Could you check a few things on this model? Use its own coordinates, in mm. A direction names the side the tool comes from. Give positions to 0.01 mm unless a question says otherwise; leave off trailing zeros. Write each loop counter-clockwise with the first axis right and the second up, starting at its lowest first coordinate (ties: lowest second). Pieces come first, ordered by that corner, then holes. Notation, with made-up numbers: M 30,89 L 61,89 A27 ccw 61,121 Z; hole C 9,47.25 d8. An arc over 180 degrees is marked long. One line per item, written item: value.
```python
from build123d import *

# Parameters (mm, degrees)
SKETCH1_R           = 10
BOSS_EXTRUDE1_DEPTH = 6
BOSS_EXTRUDE2_DEPTH = 6
CIRPATTERN1_COUNT   = 24
SKETCH3_R           = 12.65
SKETCH3_R_2         = 12
CUT_EXTRUDE1_DEPTH  = 6
CUT_EXTRUDE2_DEPTH  = 6
SKETCH5_R           = 1.5
CUT_EXTRUDE3_DEPTH  = 6
BOSS_EXTRUDE3_DEPTH = 6


with BuildPart() as part:
    # Sketch1 → Boss-Extrude1 (new body)
    with BuildSketch(Plane.XY):
        Circle(SKETCH1_R)
    extrude(amount=BOSS_EXTRUDE1_DEPTH)

    # Sketch2 → Boss-Extrude2 (add)
    with BuildSketch(Plane.XY):
        with BuildLine():
            Line((0, 12.65), (-0.9, 9.959417654))
            ThreePointArc((-0.9, 9.959417654), (0, 10), (0.9, 9.959417654))
            Line((0.9, 9.959417654), (0, 12.65))
        make_face()
    boss_extrude2 = extrude(amount=BOSS_EXTRUDE2_DEPTH)

    # CirPattern1: Boss-Extrude2 ×24 about axis
    cirpattern1_axis = Axis((0, 0, 0), (0, 0, 1))
    for i in range(1, CIRPATTERN1_COUNT):
        add(boss_extrude2.rotate(cirpattern1_axis, i * 360 / CIRPATTERN1_COUNT))

    # Sketch3 → Cut-Extrude1 (cut)
    with BuildSketch(Plane.XY):
        Circle(SKETCH3_R)
        Circle(SKETCH3_R_2, mode=Mode.SUBTRACT)
    extrude(amount=CUT_EXTRUDE1_DEPTH, mode=Mode.SUBTRACT)

    # Sketch4 → Cut-Extrude2 (cut)
    with BuildSketch(Plane.XY):
        with BuildLine():
            Line((0, 0), (0, 12))
            ThreePointArc((0, 12), (11.769423365, -2.341083864), (-4.592201188, -11.08655439))
            Line((-4.592201188, -11.08655439), (-3.826834324, -9.238795325))
            Line((-3.826834324, -9.238795325), (0, 0))
        make_face()
    extrude(amount=CUT_EXTRUDE2_DEPTH, mode=Mode.SUBTRACT)

    # Sketch5 → Cut-Extrude3 (cut)
    with BuildSketch(Plane.XY):
        Circle(SKETCH5_R)
    extrude(amount=CUT_EXTRUDE3_DEPTH, mode=Mode.SUBTRACT)

    # Sketch6 → Boss-Extrude3 (add)
    with BuildSketch(Plane.XY):
        with BuildLine():
            Line((0, 1.5), (0, 12))
            Line((0, 12), (7, 12))
            Line((7, 12), (7, 9.904493766))
            Line((7, 9.904493766), (11, 9.904493766))
            Line((11, 9.904493766), (11, -10.095506234))
            Line((11, -10.095506234), (7, -10.095506234))
            Line((7, -10.095506234), (7, -13.095506234))
            Line((7, -13.095506234), (0, -13.095506234))
            Line((0, -13.095506234), (0, -10.095506234))
            Line((0, -10.095506234), (-3.826834324, -10.095506234))
            Line((-3.826834324, -10.095506234), (-3.826834324, -9.238795325))
            Line((-3.826834324, -9.238795325), (-0.574025149, -1.385819299))
            ThreePointArc((-0.574025149, -1.385819299), (1.471177921, -0.292635483), (0, 1.5))
        make_face()
    extrude(amount=BOSS_EXTRUDE3_DEPTH)


solid = part.part
```
1) We'd pull the mould along Y, two halves only. Please class faces 1 (the face through (7, -12, 3)), 2 (the face through (-2.293, 10.737, 2.958)), 3 (the face through (-9.777, -4.994, 2.958)): pulls with the +Y half, pulls with the -Y half, needs draft (parallel to the pull), parting line crosses it, or undercut.
Outcome:
face 1: needs draft
face 2: pulls with the +Y half
face 3: undercut
2) If we section it at B-B, the plane x = -2.25: Write out the boundary of the cut face in (y, z).
Outcome:
outline: M -10.1,0 L 10.67,0 L 10.67,6 L -10.1,6 Z
3) I'm going to push flat-ended pins straight in: pin 1 (2.5 mm diameter, centred on y = 11.5, z = 4, fed in from +X); pin 2 (1.2 mm diameter, centred on x = 9.5, z = 4, fed in from +Y); pin 3 (2 mm diameter, centred on x = 8.5, z = 4.5, fed in from -Y); pin 4 (5 mm diameter, centred on x = 0, y = 0, fed in from -Z). Where does each tip first touch, or does it pass through?
Outcome:
pin 1: stops at x = 7
pin 2: stops at y = 9.9
pin 3: stops at y = -10.1
pin 4: stops at z = 0
4) On a 3-axis mill with a long thin cutter (end or side, diameter ignored), from which of +Z, -Z, +X, -X, +Y, -Y can I reach the whole of each face in a straight line? I mean faces 4 (the face through (9, 9.904, 3)), 5 (the face through (-5.977, 9.243, 2.958)), 6 (the face through (-10.993, -0.554, 2.958)), 7 (the face through (3, 12, 3)), 8 (the face through (-1.3, 9.915, 2.958)). Say none if no direction works.
Outcome:
face 4: +Z, -Z, +X, +Y
face 5: +Z, -Z
face 6: +Z, -Z, -X
face 7: +Z, -Z, +X, -X, +Y
face 8: +Z, -Z, +Y
5) Please list where these lines run through material, in increasing order: L1, parallel to X at y = 0, z = 3.2; L2, parallel to Y at x = -11, z = 4.8; L3, parallel to X at y = 9.5, z = 3.4. Write a range as from..to.
Outcome:
L1: x = -12..-1.5, 1.5..11
L2: y = -3.35..-2.47, -0.55..0.55, 2.47..3.35
L3: x = -6.03..-4.68, -3.44..11
6) If we section it at A-A, the plane x = 8.25: Write out the boundary of the cut face in (y, z).
Outcome:
outline: M -10.1,0 L 9.9,0 L 9.9,6 L -10.1,6 Z
